Here's how the part is built. I have some questions about the finished solid (model axes, mm). A direction names the side the tool comes from. Round coordinates to 2 decimals unless told otherwise and drop trailing zeros. Order: outer loops, then holes, each group sorted by start corner. A loop starts at its lowest first (then second) coordinate and runs counter-clockwise, first axis right, second up. Notation, with made-up numbers: (-32.5, 19.5) - (-14.5, 19.5) arc R16 cw to (-14.5, 49.5) - close; hole circle Ø11 at (63, 82.5). An arc over 180 degrees is marked (long way). Answer as a JSON object with one key per item and string values.
```python
from build123d import *

# Parameters (mm, degrees)
SKETCH1_W          = 25.4
SKETCH1_H          = 25.4
SKETCH1_W_2        = 19.05
SKETCH1_H_2        = 19.05
EXTRUDE1_DEPTH     = 50.8
SKETCH2_R          = 3.175
CUT_EXTRUDE1_DEPTH = 26.4
SKETCH3_R          = 3.175
CUT_EXTRUDE2_DEPTH = 26.4


with BuildPart() as part:
    # Sketch1 → Extrude1 (new body)
    with BuildSketch(Plane(origin=(0, 0, 0), x_dir=(0, 0, -1), z_dir=(1, 0, 0))):
        with Locations((12.7, 12.7)):
            Rectangle(SKETCH1_W, SKETCH1_H)
        with Locations((12.7, 12.7)):
            Rectangle(SKETCH1_W_2, SKETCH1_H_2, mode=Mode.SUBTRACT)
    extrude(amount=EXTRUDE1_DEPTH)

    # Sketch2 → Cut-Extrude1 (cut, through all)
    with BuildSketch(Plane.XY):
        with Locations((25.4, 12.7)):
            Circle(SKETCH2_R)
    extrude(amount=-CUT_EXTRUDE1_DEPTH, mode=Mode.SUBTRACT)

    # Sketch3 → Cut-Extrude2 (cut, through all)
    with BuildSketch(Plane(origin=(0, 25.4, 0), x_dir=(-1, 0, 0), z_dir=(0, 1, 0))):
        with Locations((-38.1, -12.7)):
            Circle(SKETCH3_R)
        with Locations((-12.7, -12.7)):
            Circle(SKETCH3_R)
    extrude(amount=-CUT_EXTRUDE2_DEPTH, mode=Mode.SUBTRACT)


solid = part.part
```
1. Thinking about a two-plate mould opening in X: for faces 3 (the face through (0, 13, -24)), 4 (the face through (28.33, 11.48, -23.79)), 5 (the face through (25, 0, -13)), which applies, pulls with the +X half, pulls with the -X half, needs draft (parallel to the pull), parting line crosses it, or undercut?
Responses:
{"face 3": "pulls with the -X half", "face 4": "undercut", "face 5": "needs draft"}
2. Imagine slicing it at A-A (z = -20.75). List the corners of the cut face in (x, y) for me (3 decimals).
Responses:
{"outline": "(0, 0) - (50.8, 0) - (50.8, 3.175) - (0, 3.175) - close; (0, 22.225) - (50.8, 22.225) - (50.8, 25.4) - (0, 25.4) - close"}
3. For faces 1 (the face through (28.33, 11.48, -1.57)), 2 (the face through (25, 22.225, -13)), which set-ups out of +Z, -Z, +X, -X, +Y, -Y let a thin tool reach every point of the face, with its end or its side?
Responses:
{"face 1": "+Z, -Z", "face 2": "+X, -X"}
4. Imagine slicing it at B-B (x = 45). List the corners of the cut face in (y, z) for me (3 decimals).
Responses:
{"outline": "(0, -25.4) - (25.4, -25.4) - (25.4, 0) - (0, 0) - close; hole (3.175, -22.225) - (22.225, -22.225) - (22.225, -3.175) - (3.175, -3.175) - close"}
5. Imagine slicing it at C-C (z = -12.7). List the corners of the cut face in (x, y) for me (3 decimals).
Responses:
{"outline": "(0, 0) - (9.525, 0) - (9.525, 3.175) - (0, 3.175) - close; (0, 22.225) - (9.525, 22.225) - (9.525, 25.4) - (0, 25.4) - close; (15.875, 0) - (34.925, 0) - (34.925, 3.175) - (15.875, 3.175) - close; (15.875, 22.225) - (34.925, 22.225) - (34.925, 25.4) - (15.875, 25.4) - close; (41.275, 0) - (50.8, 0) - (50.8, 3.175) - (41.275, 3.175) - close; (41.275, 22.225) - (50.8, 22.225) - (50.8, 25.4) - (41.275, 25.4) - close"}
6. Imagine slicing it at D-D (y = 12.7). List the corners of the cut face in (x, z) for me (3 decimals).
Responses:
{"outline": "(0, -25.4) - (22.225, -25.4) - (22.225, -22.225) - (0, -22.225) - close; (0, -3.175) - (22.225, -3.175) - (22.225, 0) - (0, 0) - close; (28.575, -25.4) - (50.8, -25.4) - (50.8, -22.225) - (28.575, -22.225) - close; (28.575, -3.175) - (50.8, -3.175) - (50.8, 0) - (28.575, 0) - close"}
7. For P1, Ø5.5, axis at x = 25.4, y = 12.7, coming from the +Z side, with a flat end and sliding along its axis, tell me the tip position at first contact or that it passes through.
Responses:
{"P1": "through"}
8. If I drill on L1, parallel to Z at x = 12.7, y = 1.15 (3 decimals); L2, parallel to Y at x = 25.4, z = -23.9 (3 decimals); L3, parallel to Z at x = 18, y = 17.25 (3 decimals), over which ranges is the centre line in solid material (lowest first)? Write a range as [from, to].
Responses:
{"L1": "[-25.4, -15.875], [-9.525, 0]", "L2": "[0, 9.525], [15.875, 25.4]", "L3": "[-25.4, -22.225], [-3.175, 0]"}
